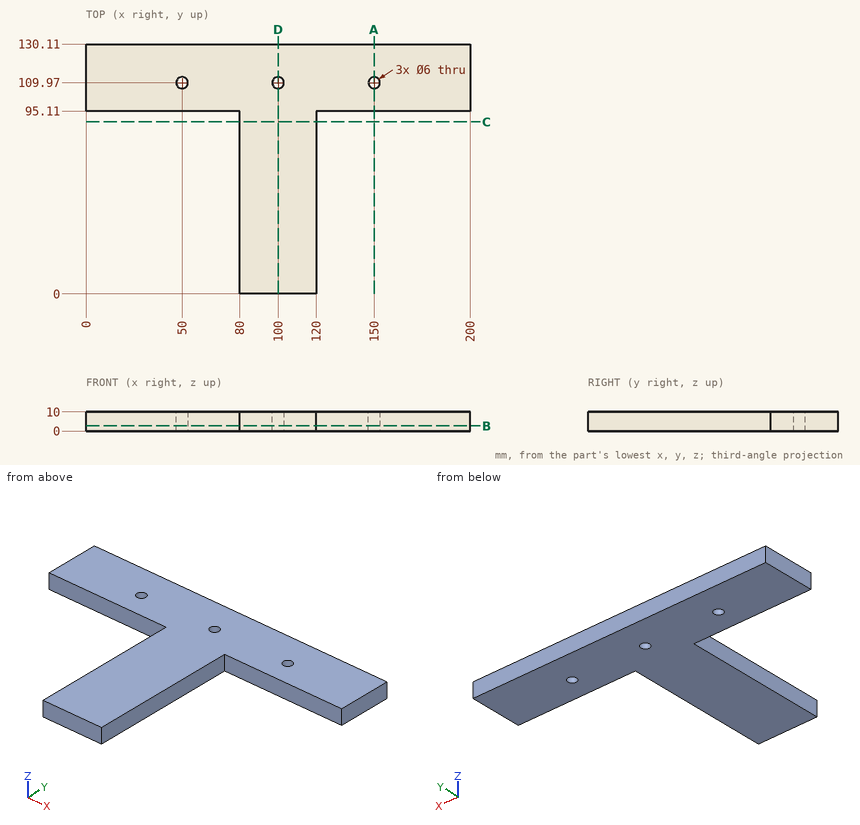
The figure shows three views and two pictorial views of one solid part (mm, origin at its lowest corner). Answer the questions. Give positions to 0.01 mm unless a question says otherwise; leave off trailing zeros. Order: outer loops, then holes, each group sorted by start corner. A loop starts at its lowest first (then second) coordinate and runs counter-clockwise, first axis right, second up. Notation, with made-up numbers: M 84.25,-6.75 L 120.25,-6.75 A20 ccw 120.25,10.25 Z; hole C 69.5,25 d9. An arc over 180 degrees is marked long. Return JSON: item names as keys, results as strings.
1) Straight lines are drawn through the part: line 1 along X through (y, z) = (109.5, 3.5); line 2 along Y through (x, z) = (100.5, 8.5); line 3 along Y through (x, z) = (150, 6.25). For each, find the intervals that lie inside material, in ascending order. Write a range as [from, to].
Resolved:
{"line 1": "[0, 47.04], [52.96, 97.04], [102.96, 147.04], [152.96, 200]", "line 2": "[0, 107.01], [112.93, 130.11]", "line 3": "[95.11, 106.97], [112.97, 130.11]"}
2) Section A-A, the plane x = 150 is taken. Write down the section's boundary in (y, z).
Resolved:
{"outline": "M 95.11,0 L 106.97,0 L 106.97,10 L 95.11,10 Z; M 112.97,0 L 130.11,0 L 130.11,10 L 112.97,10 Z"}
3) Section D-D, the plane x = 100 is taken. Write down the section's boundary in (y, z), plus the area to 3 significant figures.
Resolved:
{"outline": "M 0,0 L 106.97,0 L 106.97,10 L 0,10 Z; M 112.97,0 L 130.11,0 L 130.11,10 L 112.97,10 Z", "area": "1,240 mm^2"}
4) Each of these flat-tipped pins is pushed along its axis until it touches: pin 1 (1.5 mm diameter, centred on x = 66.5, z = 4, fed in from -Y); pin 2 (4 mm diameter, centred on y = 17, z = 6.5, fed in from +X); pin 3 (1 mm diameter, centred on y = 80, z = 5, fed in from -X). Where does it stop, or does it pass through?
Resolved:
{"pin 1": "y = 95.11", "pin 2": "x = 120", "pin 3": "x = 80"}
5) Section B-B, the plane z = 2.75 is taken. Write down the section's boundary in (x, y).
Resolved:
{"outline": "M 0,95.11 L 80,95.11 L 80,0 L 120,0 L 120,95.11 L 200,95.11 L 200,130.11 L 0,130.11 Z; hole C 50,109.97 d6; hole C 100,109.97 d6; hole C 150,109.97 d6"}
6) Section C-C, the plane y = 89.5 is taken. Write down the section's boundary in (x, z).
Resolved:
{"outline": "M 80,0 L 120,0 L 120,10 L 80,10 Z"}
